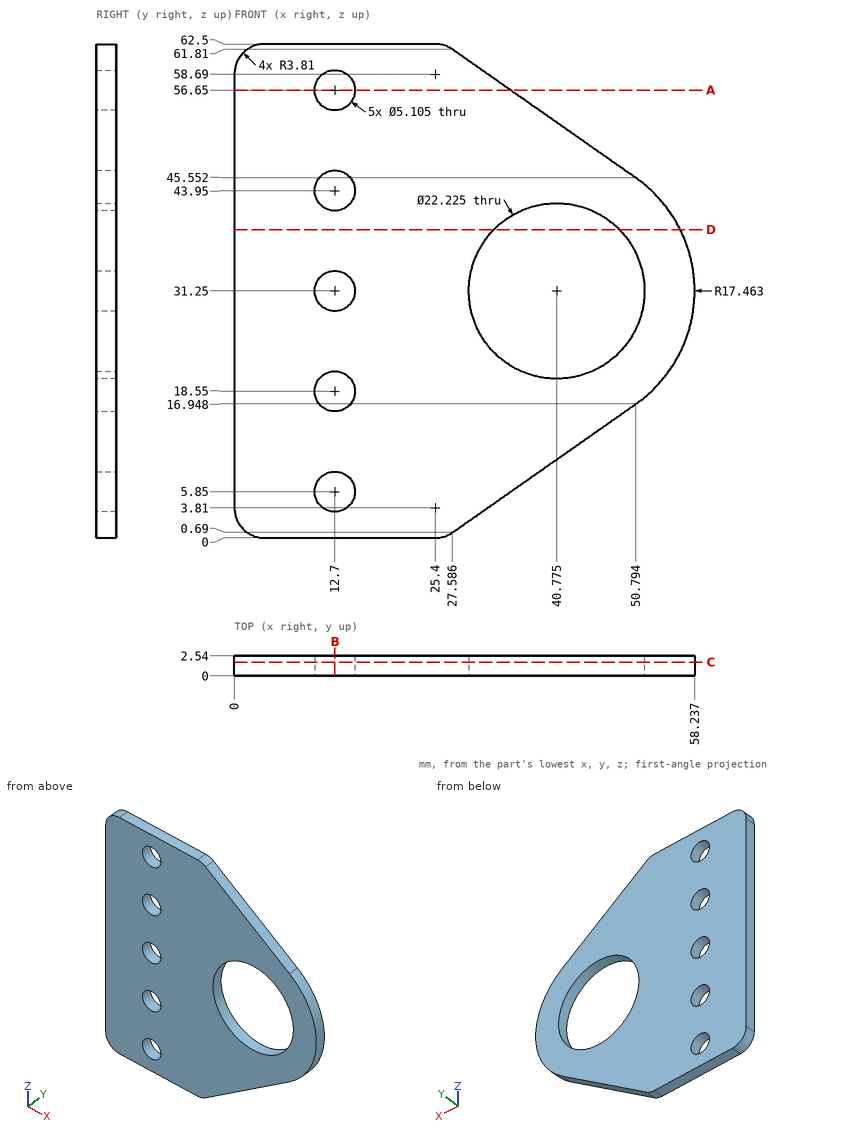
Check sheet for the drawn part. Datum: minimum x, y, z corner. Units: mm. Round coordinates to 2 decimals unless told otherwise and drop trailing zeros. Write each loop counter-clockwise with the first axis right and the second up, starting at its lowest first coordinate (ties: lowest second). Pieces come first, ordered by that corner, then holes. Notation, with made-up numbers: (66, 56.25) -> (88, 56.25) arc R28 ccw to (88, 82.25) -> close; hole circle Ø1 at (6, 27.5). An arc over 180 degrees is marked (long way). Put each result on its own line as item: value.
(1) Sectioned sample at C-C (y = 1.75). Count the separate pieces of the cut face and the enclosed holes in it, plus the area to 3 significant figures.
Values found:
separate pieces: 1
enclosed holes: 6
area: 2,420 mm^2
(2) Sectioned sample at A-A (z = 56.65). Enter the section's corners in (x, y).
Values found:
outline: (0, 0) -> (10.15, 0) -> (10.15, 2.54) -> (0, 2.54) -> close; (15.25, 0) -> (34.95, 0) -> (34.95, 2.54) -> (15.25, 2.54) -> close
(3) Sectioned sample at B-B (x = 12.7). Enter the section's corners in (y, z).
Values found:
outline: (0, 0) -> (2.54, 0) -> (2.54, 3.3) -> (0, 3.3) -> close; (0, 8.4) -> (2.54, 8.4) -> (2.54, 16) -> (0, 16) -> close; (0, 21.1) -> (2.54, 21.1) -> (2.54, 28.7) -> (0, 28.7) -> close; (0, 33.8) -> (2.54, 33.8) -> (2.54, 41.4) -> (0, 41.4) -> close; (0, 46.5) -> (2.54, 46.5) -> (2.54, 54.1) -> (0, 54.1) -> close; (0, 59.2) -> (2.54, 59.2) -> (2.54, 62.5) -> (0, 62.5) -> close
(4) Go/stop test with a flat-tipped pin: pin 1 Ø6.5 at (x, z) = (12.7, 56.65) entering from -Y. Record where the tip stops, or that it passes through.
Values found:
pin 1: stops at y = 0
(5) Sectioned sample at D-D (z = 39). Enter the section's corners in (x, y), plus the area to 3 significant figures.
Values found:
outline: (0, 0) -> (32.81, 0) -> (32.81, 2.54) -> (0, 2.54) -> close; (48.74, 0) -> (56.42, 0) -> (56.42, 2.54) -> (48.74, 2.54) -> close
area: 103 mm^2
(6) Material ranges on line 1 (X direction, y = 0.7, z = 31.5) (1 decimal); line 2 (Z direction, x = 35, y = 0.15) (1 decimal); line 3 (X direction, y = 0.95, z = 30) (1 decimal), recorded low to high.
Values found:
line 1: x = 0 to 10.2, 15.2 to 29.7, 51.9 to 58.2
line 2: z = 5.9 to 21.8, 40.7 to 56.6
line 3: x = 0 to 10.5, 14.9 to 29.7, 51.8 to 58.2
